For this review, take the finished solid that the model builds, in its own axes (mm). Coordinates: 2 decimals unless noted, no trailing zeros. Loops run counter-clockwise (first coordinate to the right, second up) from the corner with the lowest first, then second, coordinate; pieces in that order, holes last. Notation, with made-up numbers: (65.25, 85.25) -> (96.25, 85.25) arc R29 cw to (96.25, 111.25) -> close; hole circle Ø11 at (64, 88.5). An arc over 180 degrees is marked (long way). Use a Markdown table: item, result.
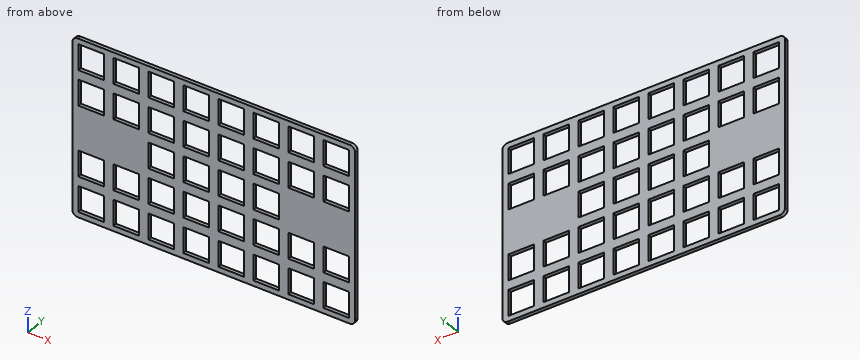
from build123d import *

# Parameters (mm, degrees)
BOSS_EXTRUDE1_DEPTH     = 2
CUT_EXTRUDE3_DEPTH      = 178.128669687
CUT_EXTRUDE3_DEPTH_BACK = 178.128669687
SKETCH14_W              = 14
SKETCH14_H              = 14


with BuildPart() as part:
    # Sketch16 → Boss-Extrude1 (new body)
    with BuildSketch(Plane(origin=(0, 0, 0), x_dir=(1, 0, 0), z_dir=(0, 1, 0))):
        with BuildLine():
            Line((-0.325, 93.1), (147.675, 93.1))
            ThreePointArc((147.675, 93.1), (149.796320344, 92.221320344), (150.675, 90.1))
            Line((150.675, 90.1), (150.675, 0.1))
            ThreePointArc((150.675, 0.1), (149.796320344, -2.021320344), (147.675, -2.9))
            Line((147.675, -2.9), (-0.325, -2.9))
            ThreePointArc((-0.325, -2.9), (-2.446320344, -2.021320344), (-3.325, 0.1))
            Line((-3.325, 0.1), (-3.325, 90.1))
            ThreePointArc((-3.325, 90.1), (-2.446320344, 92.221320344), (-0.325, 93.1))
        make_face()
    extrude(amount=BOSS_EXTRUDE1_DEPTH)

    # Sketch14 → Cut-Extrude3 (cut, two sides: drawn at the far end of the back side and taken through both)
    with BuildSketch(Plane(origin=(0, 0, 0), x_dir=(1, 0, 0), z_dir=(0, 1, 0)).offset(-CUT_EXTRUDE3_DEPTH_BACK)):
        with Locations((26.05, 7)):
            Rectangle(SKETCH14_W, SKETCH14_H)
        with Locations((7, 7)):
            Rectangle(SKETCH14_W, SKETCH14_H)
        with Locations((45.1, 7)):
            Rectangle(SKETCH14_W, SKETCH14_H)
        with Locations((64.15, 7)):
            Rectangle(SKETCH14_W, SKETCH14_H)
        with Locations((83.2, 7)):
            Rectangle(SKETCH14_W, SKETCH14_H)
        with Locations((102.25, 7)):
            Rectangle(SKETCH14_W, SKETCH14_H)
        with Locations((121.3, 7)):
            Rectangle(SKETCH14_W, SKETCH14_H)
        with Locations((140.35, 7)):
            Rectangle(SKETCH14_W, SKETCH14_H)
        with Locations((26.05, 26.05)):
            Rectangle(SKETCH14_W, SKETCH14_H)
        with Locations((45.1, 26.05)):
            Rectangle(SKETCH14_W, SKETCH14_H)
        with Locations((64.15, 26.05)):
            Rectangle(SKETCH14_W, SKETCH14_H)
        with Locations((83.2, 26.05)):
            Rectangle(SKETCH14_W, SKETCH14_H)
        with Locations((102.25, 26.05)):
            Rectangle(SKETCH14_W, SKETCH14_H)
        with Locations((121.3, 26.05)):
            Rectangle(SKETCH14_W, SKETCH14_H)
        with Locations((140.35, 26.05)):
            Rectangle(SKETCH14_W, SKETCH14_H)
        with Locations((45.1, 45.1)):
            Rectangle(SKETCH14_W, SKETCH14_H)
        with Locations((64.15, 45.1)):
            Rectangle(SKETCH14_W, SKETCH14_H)
        with Locations((83.2, 45.1)):
            Rectangle(SKETCH14_W, SKETCH14_H)
        with Locations((102.25, 45.1)):
            Rectangle(SKETCH14_W, SKETCH14_H)
        with Locations((26.05, 64.15)):
            Rectangle(SKETCH14_W, SKETCH14_H)
        with Locations((45.1, 64.15)):
            Rectangle(SKETCH14_W, SKETCH14_H)
        with Locations((64.15, 64.15)):
            Rectangle(SKETCH14_W, SKETCH14_H)
        with Locations((83.2, 64.15)):
            Rectangle(SKETCH14_W, SKETCH14_H)
        with Locations((102.25, 64.15)):
            Rectangle(SKETCH14_W, SKETCH14_H)
        with Locations((121.3, 64.15)):
            Rectangle(SKETCH14_W, SKETCH14_H)
        with Locations((140.35, 64.15)):
            Rectangle(SKETCH14_W, SKETCH14_H)
        with Locations((26.05, 83.2)):
            Rectangle(SKETCH14_W, SKETCH14_H)
        with Locations((45.1, 83.2)):
            Rectangle(SKETCH14_W, SKETCH14_H)
        with Locations((64.15, 83.2)):
            Rectangle(SKETCH14_W, SKETCH14_H)
        with Locations((83.2, 83.2)):
            Rectangle(SKETCH14_W, SKETCH14_H)
        with Locations((102.25, 83.2)):
            Rectangle(SKETCH14_W, SKETCH14_H)
        with Locations((121.3, 83.2)):
            Rectangle(SKETCH14_W, SKETCH14_H)
        with Locations((140.35, 83.2)):
            Rectangle(SKETCH14_W, SKETCH14_H)
        with Locations((7, 26.05)):
            Rectangle(SKETCH14_W, SKETCH14_H)
        with Locations((7, 64.15)):
            Rectangle(SKETCH14_W, SKETCH14_H)
        with Locations((7, 83.2)):
            Rectangle(SKETCH14_W, SKETCH14_H)
    extrude(amount=CUT_EXTRUDE3_DEPTH + CUT_EXTRUDE3_DEPTH_BACK, mode=Mode.SUBTRACT)


solid = part.part
(1) Take a section at B-B on z = -48.5. Write out the cut boundary in (x, y) (3 decimals), plus the area to 3 significant figures.
Found:
| item | result |
|---|---|
| outline | (-3.325, 0) -> (38.1, 0) -> (38.1, 2) -> (-3.325, 2) -> close; (52.1, 0) -> (57.15, 0) -> (57.15, 2) -> (52.1, 2) -> close; (71.15, 0) -> (76.2, 0) -> (76.2, 2) -> (71.15, 2) -> close; (90.2, 0) -> (95.25, 0) -> (95.25, 2) -> (90.2, 2) -> close; (109.25, 0) -> (150.675, 0) -> (150.675, 2) -> (109.25, 2) -> close |
| area | 196 mm^2 |
(2) For line 1 along Z through (x, y) = (44, 1.5); line 2 along Z through (x, y) = (28, 0.6); line 3 along X through (y, z) = (1.5, -39) (3 decimals), list the stretches that pass through material, from the lowest coordinate up.
Found:
| item | result |
|---|---|
| line 1 | z = -93.1 to -90.2, -76.2 to -71.15, -57.15 to -52.1, -38.1 to -33.05, -19.05 to -14, 0 to 2.9 |
| line 2 | z = -93.1 to -90.2, -76.2 to -71.15, -57.15 to -33.05, -19.05 to -14, 0 to 2.9 |
| line 3 | x = -3.325 to 38.1, 52.1 to 57.15, 71.15 to 76.2, 90.2 to 95.25, 109.25 to 150.675 |
(3) Take a section at A-A on x = 122.5. Write out the cut boundary in (y, z).
Found:
| item | result |
|---|---|
| outline | (0, -93.1) -> (2, -93.1) -> (2, -90.2) -> (0, -90.2) -> close; (0, -76.2) -> (2, -76.2) -> (2, -71.15) -> (0, -71.15) -> close; (0, -57.15) -> (2, -57.15) -> (2, -33.05) -> (0, -33.05) -> close; (0, -19.05) -> (2, -19.05) -> (2, -14) -> (0, -14) -> close; (0, 0) -> (2, 0) -> (2, 2.9) -> (0, 2.9) -> close |
(4) Take a section at C-C on z = -4.5. State how many separate pieces and enclosed holes the cut face has, plus the area to 3 significant figures.
Found:
| item | result |
|---|---|
| separate pieces | 9 |
| enclosed holes | 0 |
| area | 84.0 mm^2 |
